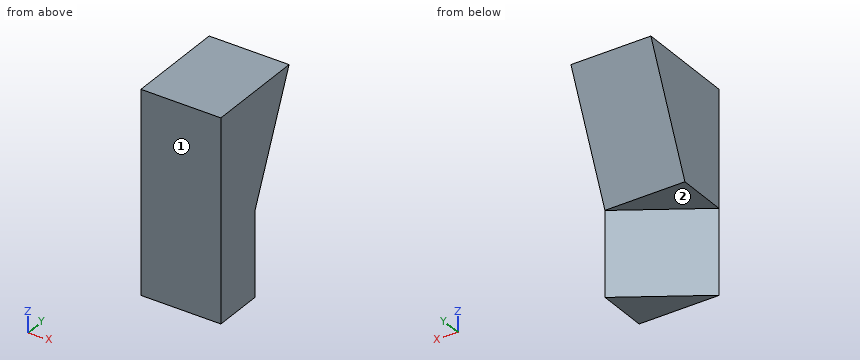
```python
from build123d import *

# Parameters (mm, degrees)
SKETCH2_W           = 40
SKETCH2_H           = 5
SKETCH2_W_2         = 5
SKETCH2_H_2         = 100
BOSS_EXTRUDE1_DEPTH = 30
SKETCH3_W           = 3
SKETCH3_H           = 3
CUT_EXTRUDE1_DEPTH  = 5
SKETCH2_4_W         = 40
SKETCH2_4_H         = 100
BOSS_EXTRUDE2_DEPTH = 5
CUT_EXTRUDE2_DEPTH  = 25
BOSS_EXTRUDE3_DEPTH = 25
SKETCH10_W          = 40
SKETCH10_H          = 5
BOSS_EXTRUDE4_DEPTH = 35
SKETCH11_W          = 5
SKETCH11_H          = 5
CUT_EXTRUDE5_DEPTH  = 6
SKETCH11_4_W        = 5
SKETCH11_4_H        = 5
CUT_EXTRUDE6_DEPTH  = 4.99
BOSS_EXTRUDE5_DEPTH = 50
SKETCH12_3_W        = 40
SKETCH12_3_H        = 42.17911114
BOSS_EXTRUDE6_DEPTH = 25
CHAMFER1_SIZE       = 25.021332939
CHAMFER1_SIZE_2     = 57.82088886
CUT_EXTRUDE7_DEPTH  = 42.2284
SKETCH15_W          = 50
SKETCH15_H          = 110
CUT_EXTRUDE8_DEPTH  = 40
SKETCH16_W          = 40
SKETCH16_H          = 100
SKETCH16_W_2        = 39.6
SKETCH16_H_2        = 99.6
CUT_EXTRUDE9_DEPTH  = 50


with BuildPart() as part:
    # Sketch2 → Boss-Extrude1 (new body)
    with BuildSketch(Plane(origin=(0, 0, 0), x_dir=(1, 0, 0), z_dir=(0, 1, 0))):
        Polygon((-22.5, 60), (-22.5, -50), (-17.5, -50), (-17.5, -45), (-17.5, 55), (-17.5, 60), align=None)
        with Locations((2.5, 57.5)):
            Rectangle(SKETCH2_W, SKETCH2_H)
        with Locations((25, 57.5)):
            Rectangle(SKETCH2_W_2, SKETCH2_H)
        with Locations((25, 5)):
            Rectangle(SKETCH2_W_2, SKETCH2_H_2)
        with Locations((25, -47.5)):
            Rectangle(SKETCH2_W_2, SKETCH2_H)
        with Locations((2.5, -47.5)):
            Rectangle(SKETCH2_W, SKETCH2_H)
    extrude(amount=-BOSS_EXTRUDE1_DEPTH)

    # Sketch3 → Cut-Extrude1 (cut)
    with BuildSketch(Plane.ZY.offset(22.5)):
        Polygon((-35, -25), (-35, -28), (-32, -28), (-32, -22), (-38, -22), (-38, -25), align=None)
        with Locations((-36.5, -26.5)):
            Rectangle(SKETCH3_W, SKETCH3_H)
    extrude(amount=-CUT_EXTRUDE1_DEPTH, mode=Mode.SUBTRACT)

    # Sketch2<4> → Boss-Extrude2 (add)
    with BuildSketch(Plane(origin=(0, 0, 0), x_dir=(1, 0, 0), z_dir=(0, 1, 0))):
        with Locations((2.5, 5)):
            Rectangle(SKETCH2_4_W, SKETCH2_4_H)
    extrude(amount=-BOSS_EXTRUDE2_DEPTH)

    # Sketch5 → Cut-Extrude2 (cut)
    with BuildSketch(Plane.XZ.offset(30)):
        Polygon((27.5, 50), (-22.5, 50), (-22.5, 45), (-17.5, 45), (17.5, 45), (22.5, 45), (22.5, -55), (17.5, -55), (-17.5, -55), (-22.5, -55), (-22.5, -60), (27.5, -60), align=None)
    extrude(amount=-CUT_EXTRUDE2_DEPTH, mode=Mode.SUBTRACT)

    # Sketch5<3> → Boss-Extrude3 (add)
    with BuildSketch(Plane.XZ.offset(30)):
        Polygon((17.5, 45), (-17.5, 45), (-17.5, 40), (12.5, 40), (12.5, -50), (-17.5, -50), (-17.5, -55), (17.5, -55), align=None)
    extrude(amount=-BOSS_EXTRUDE3_DEPTH)

    # Sketch10 → Boss-Extrude4 (add)
    with BuildSketch(Plane.XZ.offset(5)):
        with Locations((-2.5, 47.5)):
            Rectangle(SKETCH10_W, SKETCH10_H)
        with Locations((-2.5, -57.5)):
            Rectangle(SKETCH10_W, SKETCH10_H)
    extrude(amount=BOSS_EXTRUDE4_DEPTH)

    # Sketch11 → Cut-Extrude5 (cut)
    with BuildSketch(Plane(origin=(0, 0, 0), x_dir=(1, 0, 0), z_dir=(0, 1, 0))):
        with Locations((25, 52.5)):
            Rectangle(SKETCH11_W, SKETCH11_H)
        Polygon((27.5, 7.5), (22.5, 7.5), (22.5, 5), (22.5, 2.5), (27.5, 2.5), (27.5, 5), align=None)
        Polygon((27.5, -45), (27.5, -40), (24, -40), (23.5, -40), (22.5, -40), (22.5, -41), (22.5, -41.5), (22.5, -45), align=None)
    extrude(amount=-CUT_EXTRUDE5_DEPTH, mode=Mode.SUBTRACT)

    # Sketch11<4> → Cut-Extrude6 (cut)
    with BuildSketch(Plane(origin=(0, 0, 0), x_dir=(1, 0, 0), z_dir=(0, 1, 0))):
        Polygon((-17.5, 7.5), (-22.5, 7.5), (-22.5, 5), (-22.5, 2.5), (-17.5, 2.5), align=None)
        with Locations((-20, -42.5)):
            Rectangle(SKETCH11_4_W, SKETCH11_4_H)
    extrude(amount=-CUT_EXTRUDE6_DEPTH, mode=Mode.SUBTRACT)

    # Sketch12 → Boss-Extrude5 (add)
    with BuildSketch(Plane(origin=(0, 0, 0), x_dir=(1, 0, 0), z_dir=(0, 1, 0))):
        Polygon((22.5, 12.82088886), (-17.5, 12.82088886), (-17.5, 7.5), (-17.5, 2.5), (-17.5, -40), (-17.5, -45), (22.5, -45), (22.5, -40), (22.5, 2.5), (22.5, 7.5), align=None)
    extrude(amount=BOSS_EXTRUDE5_DEPTH)

    # Sketch12<3> → Boss-Extrude6 (add)
    with BuildSketch(Plane(origin=(0, 0, 0), x_dir=(1, 0, 0), z_dir=(0, 1, 0))):
        with Locations((2.5, 33.91044443)):
            Rectangle(SKETCH12_3_W, SKETCH12_3_H)
    extrude(amount=BOSS_EXTRUDE6_DEPTH)

    # Chamfer1
    # the kernel refuses this chamfer: 57.82088886, 25.021332939 mm, written as the material it takes off along each edge
    with BuildSketch(Plane(origin=(172.37635383, 50, -12.82088886), x_dir=(0, -0.9966687843763375, -0.08155571255156512), z_dir=(-1, 0, 0))) as chamfer1_piece_1_section:
        Polygon((CHAMFER1_SIZE * 0.996668784369, CHAMFER1_SIZE * 0.081555712551), (-CHAMFER1_SIZE_2 * 0.0815557125516, CHAMFER1_SIZE_2 * 0.996668784376), (0, 0), align=None)
    chamfer1_piece_1 = extrude(amount=339.752707661, mode=Mode.PRIVATE)
    chamfer1_piece_1 = split(chamfer1_piece_1, bisect_by=Plane(origin=(2.5, 25, 6.452754758), z_dir=(0, 1, 0)), keep=Keep.TOP, mode=Mode.PRIVATE)
    add(chamfer1_piece_1, mode=Mode.SUBTRACT)

    # Sketch14 → Cut-Extrude7 (cut)
    with BuildSketch(Plane(origin=(0, 0, -55), x_dir=(-1, 0, 0), z_dir=(0, 0, -1))):
        Polygon((-22.5, 25), (17.5, 0), (17.5, 25), align=None)
    extrude(amount=-CUT_EXTRUDE7_DEPTH, mode=Mode.SUBTRACT)

    # Sketch15 → Cut-Extrude8 (cut)
    with BuildSketch(Plane.XZ.offset(40)):
        with Locations((2.5, -5)):
            Rectangle(SKETCH15_W, SKETCH15_H)
    extrude(amount=-CUT_EXTRUDE8_DEPTH, mode=Mode.SUBTRACT)

    # Sketch16 → Cut-Extrude9 (cut)
    with BuildSketch(Plane.XZ):
        with Locations((2.5, -5)):
            Rectangle(SKETCH16_W, SKETCH16_H)
        with Locations((2.5, -5)):
            Rectangle(SKETCH16_W_2, SKETCH16_H_2, mode=Mode.SUBTRACT)
    extrude(amount=-CUT_EXTRUDE9_DEPTH, mode=Mode.SUBTRACT)


solid = part.part
```
CAD build for the part. Positions are in the model's coordinates, mm. Face numbers are marked on the shaded views. A direction names the side the tool comes from. Coordinates: 2 decimals unless noted, no trailing zeros. Loops run counter-clockwise (first coordinate to the right, second up) from the corner with the lowest first, then second, coordinate; pieces in that order, holes last. Notation, with made-up numbers: (53.5, 39) - (59.5, 39) arc R17 ccw to (59.5, 55) - close; hole circle Ø2 at (24.5, 1.25). An arc over 180 degrees is marked (long way). Use CSV: the item, a comma, the result in double quotes. Start each with the question number.
Q1. Cut at C-C, the plane z = -39. List the corners of the cut face in (x, y) (3 decimals).
Q2. Drop flat-ended pins along their axis: P1, Ø4, axis at x = -1.5, y = 31.5, coming from the -Z side; P2, Ø1, axis at y = 14, z = -39.5, coming from the -X side; P3, Ø3, axis at x = -4.5, z = -29.5, coming from the +Y side. Give the stop position or say it passes through.
Q3. Cut at A-A, the plane y = 16. List the corners of the cut face in (x, z).
Q4. Probe probe 1 along Z at (x, y) = (-4, 9); probe 2 along Y at (x, z) = (4, -30); probe 3 along Y at (x, z) = (9.5, -48) (3 decimals). List the from-to ranges inside material, lowest first. Write a range as from..to.
Q5. 3-axis set-ups, long thin cutter, end or side, ignore diameter. For the marked faces 1 and 2: which of +Z, -Z, +X, -X, +Y, -Y reach the whole face in a straight line?
Here are the results:
1,outline,"(-17.3, 0) - (22.3, 0) - (22.3, 24.875) - (-17.3, 0.125) - close"
2,P1,"z = -2.37"
2,P2,"x = 4.1"
2,P3,"y = 9.06"
3,outline,"(-17.3, -12.77) - (8.1, -12.77) - (8.1, -54.8) - (22.3, -54.8) - (22.3, 44.8) - (-17.3, 44.8) - close"
4,probe 1,"-12.77..44.8"
4,probe 2,"0..13.44"
4,probe 3,"0..16.875"
5,face 1,"+Z, -Z, +X, -X, -Y"
5,face 2,"-Z, -X, +Y"
